Geometry check sheet. Reference: the model listing, model coordinates, mm. A direction names the side the tool comes from. Coordinates: 2 decimals unless noted, no trailing zeros. Order: outer loops, then holes, each group sorted by start corner. A loop starts at its lowest first (then second) coordinate and runs counter-clockwise, first axis right, second up. Notation, with made-up numbers: (59.25, 45.25) - (103.25, 45.25) arc R25 cw to (103.25, 78.25) - close; hole circle Ø2 at (-34.75, -15.75). An arc over 180 degrees is marked (long way). One line per item, written item: value. Start each with the question number.
Autodesk Inventor part; units mm, degrees
ref_plane "YZ Plane" through (0, 0, 0) normal (1, 0, 0) x (0, 1, 0)
ref_plane "XZ Plane" through (0, 0, 0) normal (0, 1, 0) x (-1, 0, 0)
ref_plane "XY Plane" through (0, 0, 0) normal (0, 0, 1) x (1, 0, 0)
sketch "スケッチ1" plane through (0, 0, 0) normal (0, 0, 1) x (1, 0, 0)
  line L0 (-59.5, -21.75) -> (59.5, -21.75) construction
  line L1 (59.5, -21.75) -> (59.5, 21.75) construction
  line L2 (59.5, 21.75) -> (-59.5, 21.75) construction
  line L3 (-59.5, 21.75) -> (-59.5, -21.75) construction
  line L4 (-59.5, -21.75) -> (59.5, 21.75) construction
  line L5 (59.5, -21.75) -> (-59.5, 21.75) construction
  line L6 (-54.5, -16.75) -> (54.5, -16.75) construction
  line L7 (54.5, -16.75) -> (54.5, 16.75) construction
  line L8 (54.5, 16.75) -> (-54.5, 16.75) construction
  line L9 (-54.5, 16.75) -> (-54.5, -16.75) construction
  line L10 (-54.5, -16.75) -> (54.5, 16.75) construction
  line L11 (54.5, -16.75) -> (-54.5, 16.75) construction
  line L12 (-33.05, 11.05) -> (-27.95, 11.05)
  line L13 (-27.95, 11.05) -> (-27.95, -4.05)
  line L14 (-27.95, -4.05) -> (-33.05, -4.05)
  line L15 (-33.05, -4.05) -> (-33.05, 11.05)
  line L16 (-28, 11) -> (-33, 11) construction
  line L17 (-33, 11) -> (-33, -4) construction
  line L18 (-33, -4) -> (-28, -4) construction
  line L19 (-28, -4) -> (-28, 11) construction
  line L20 (-30.5, 11) -> (-30.5, -4) construction
  line L21 (-33, 21) -> (-28, 21) construction
  line L22 (-28, 21) -> (-28, -14) construction
  line L23 (-28, -14) -> (-33, -14) construction
  line L24 (-33, -14) -> (-33, 21) construction
  circle A0 centre (-30.5, 17) radius 1.55
  circle A1 centre (-30.5, -10) radius 1.55
  circle A2 centre (-33.05, 10) radius 1.05
  circle A3 centre (-27.95, 10) radius 1.05
  circle A4 centre (-33.05, -3) radius 1.05
  circle A5 centre (-27.95, -3) radius 1.05
  line L25 (0, 0) -> (0, 16.75) construction
  line L26 (0, 0) -> (54.5, 0) construction
  circle A6 centre (30.5, 17) radius 1.55
  circle A7 centre (30.5, -10) radius 1.55
  circle A8 centre (27.95, 10) radius 1.05
  circle A9 centre (33.05, 10) radius 1.05
  circle A10 centre (27.95, -3) radius 1.05
  circle A11 centre (33.05, -3) radius 1.05
  line L27 (33.05, 11.05) -> (27.95, 11.05)
  line L28 (27.95, 11.05) -> (27.95, -4.05)
  line L29 (27.95, -4.05) -> (33.05, -4.05)
  line L30 (33.05, -4.05) -> (33.05, 11.05)
  line L31 (-59.5, 11.75) -> (-64.5, 11.75)
  line L32 (-64.5, 11.75) -> (-64.5, -11.75)
  line L33 (-64.5, -11.75) -> (-59.5, -11.75)
  line L34 (-59.5, 13.85) -> (-59.5, 21.75)
  line L35 (-59.5, 21.75) -> (-21.6, 21.75)
  line L36 (-19.5, 21.75) -> (-19.5, 26.75)
  line L37 (-19.5, 26.75) -> (19.5, 26.75)
  line L38 (19.5, 26.75) -> (19.5, 21.75)
  line L39 (21.6, 21.75) -> (59.5, 21.75)
  line L40 (59.5, 21.75) -> (59.5, 13.85)
  line L41 (59.5, 11.75) -> (64.5, 11.75)
  line L42 (64.5, 11.75) -> (64.5, -11.75)
  line L43 (64.5, -11.75) -> (59.5, -11.75)
  line L44 (-59.5, -13.85) -> (-59.5, -21.75)
  line L45 (-59.5, -21.75) -> (59.5, -21.75)
  line L46 (59.5, -21.75) -> (59.5, -13.85)
  arc A12 (-59.5, 11.75) -> (-59.5, 13.85) centre (-59.5, 12.8) ccw
  arc A13 (-59.5, -13.85) -> (-59.5, -11.75) centre (-59.5, -12.8) ccw
  line L47 (0, 0) -> (-54.5, 0) construction
  arc A14 (59.5, -11.75) -> (59.5, -13.85) centre (59.5, -12.8) ccw
  arc A15 (59.5, 13.85) -> (59.5, 11.75) centre (59.5, 12.8) ccw
  arc A16 (-21.6, 21.75) -> (-19.5, 21.75) centre (-20.55, 21.75) ccw
  arc A17 (19.5, 21.75) -> (21.6, 21.75) centre (20.55, 21.75) ccw
  line L48 (-56.8855, 19.3) -> (-54.5, 19.3) construction
  line L49 (-54.5, 19.3) -> (-54.5, 16.2) construction
  line L50 (-54.5, 16.2) -> (-56.8855, 16.2) construction
  line L51 (-56.8855, 16.2) -> (-56.8855, 19.3) construction
  line L52 (-54.5, 17.75) -> (-56.8855, 17.75) construction
  line L53 (-53.05, 22.7202) -> (-49.95, 22.7202) construction
  line L54 (-49.95, 22.7202) -> (-49.95, 16.75) construction
  line L55 (-49.95, 16.75) -> (-53.05, 16.75) construction
  line L56 (-53.05, 16.75) -> (-53.05, 22.7202) construction
  line L57 (-51.5, 22.7202) -> (-51.5, 16.75) construction
  point P0 (-30.5, -14)
  dimension "d10" = 2.1
  dimension "d0" = 33.5
  dimension "d1" = 5
  dimension "d2" = 109
  dimension "d3" = 5
  dimension "d4" = 0.05
  dimension "d5" = 35
  dimension "d6" = 27
  dimension "d7" = 5
  dimension "d11" = 33
  dimension "d12" = 3.1
  dimension "d13" = 1.05
  dimension "d14" = 5
  dimension "d15" = 4
  dimension "d16" = 3.1
  dimension "d17" = 10
  dimension "d18" = 5
  dimension "d19" = 8
  dimension "d20" = 5
  dimension "d21" = 40
  dimension "d22" = 5
  dimension "d50" = 4
  dimension "d51" = 10
  dimension "d52" = 17
  dimension "d53" = 10
extrude "押し出し1" add sketch "スケッチ1" along normal blind 5
sketch "スケッチ2" plane through (0, 0, 5) normal (0, 0, 1) x (1, 0, 0)
  circle A0 centre (30.5, -10) radius 1.55
  circle A1 centre (30.5, 17) radius 1.55
  circle A2 centre (-30.5, -10) radius 1.55
  circle A3 centre (-30.5, 17) radius 1.55
  point P0 (0, 0)
hole "穴1" at (-30.5, 17, 5) at (-30.5, -10, 5) at (30.5, 17, 5) at (30.5, -10, 5) direction (0, 0, -1) diameter 6 depth 3
sketch "スケッチ3" plane through (59.5, -21.75, 0) normal (1, 0, 0) x (0, 0, -1)
  line L0 (0, 0) -> (-5, 0)
  line L1 (0, 43.5) -> (-5, 43.5)
  point P0 (0, 21.75)
  point P1 (-2.5, 4)
  point P2 (-2.5, 39.5)
  point P3 (-2.5, 0)
  dimension "d32" = 4
  dimension "d33" = 4
hole "穴2" at (59.5, -17.75, 2.5) at (59.5, 17.75, 2.5) direction (-1, 0, 0) diameter 2.459 depth 2.5
mirror "ミラー1" about plane through (0, 0, 0) normal (1, 0, 0) of "穴2"
sketch "スケッチ5" plane through (0, 0, 5) normal (0, 0, 1) x (1, 0, 0)
  line L0 (27.95, -1.95) -> (27.95, 8.95)
  line L1 (-33.05, -1.95) -> (-33.05, 8.95)
  line L2 (-27.95, 8.95) -> (-27.95, -1.95)
  line L3 (-59.5, -21.75) -> (59.5, -21.75)
  line L4 (19.5, 26.75) -> (-19.5, 26.75)
  line L5 (-21.6, 21.75) -> (-59.5, 21.75)
  line L6 (-59.5, 21.75) -> (-59.5, 13.85)
  line L7 (-52.5, 14.75) -> (-38, 14.75)
  line L8 (-38, 14.75) -> (-38, -14.75)
  line L9 (-38, -14.75) -> (-52.5, -14.75)
  line L10 (-52.5, -14.75) -> (-52.5, 14.75)
  line L11 (38, 14.75) -> (52.5, 14.75)
  line L12 (52.5, 14.75) -> (52.5, -14.75)
  line L13 (52.5, -14.75) -> (38, -14.75)
  line L14 (38, -14.75) -> (38, 14.75)
  line L15 (-23, 16.75) -> (-23, -9.0978)
  line L16 (-23, -9.0978) -> (20.2083, 16.75)
  line L17 (20.2083, 16.75) -> (-23, 16.75)
  line L18 (23, 9.0978) -> (23, -16.75)
  line L19 (23, -16.75) -> (-20.2083, -16.75)
  line L20 (-20.2083, -16.75) -> (23, 9.0978)
  line L21 (-33, 9.2736) -> (-28, 9.2736) construction
  line L22 (-28, 9.2736) -> (-28, -5.1442) construction
  line L23 (-28, -5.1442) -> (-33, -5.1442) construction
  line L24 (-33, -5.1442) -> (-33, 9.2736) construction
  line L25 (0, 0) -> (0, 26.75) construction
  line L26 (28, 10.3975) -> (29.3974, 10.3975) construction
  line L27 (29.3974, 10.3975) -> (29.3974, -4.5864) construction
  line L28 (29.3974, -4.5864) -> (28, -4.5864) construction
  line L29 (28, -4.5864) -> (28, 10.3975) construction
  line L30 (28, 16.75) -> (-28, -16.75) construction
  line L31 (-28, 16.75) -> (28, 16.75) construction
  line L32 (28, 16.75) -> (28, -16.75) construction
  line L33 (28, -16.75) -> (-28, -16.75) construction
  line L34 (-28, -16.75) -> (-28, 16.75) construction
  line L35 (59.5, 21.75) -> (21.6, 21.75)
  dimension "d54" = 7
  dimension "d55" = 7
  dimension "d56" = 7
  dimension "d57" = 0.05
  dimension "d58" = 5
  dimension "d59" = 0.05
  dimension "d60" = 5
  dimension "d62" = 5
  dimension "d63" = 0.05
  dimension "d64" = 8
  dimension "d68" = 5
extrude "押し出し2" cut sketch "スケッチ5" against normal blind 10
fillet "フィレット1" radius 3 14 edges at (-38, 14.75, 2.5) (-52.5, 14.75, 2.5) (-52.5, -14.75, 2.5) (-38, -14.75, 2.5) (-23, -9.0978, 2.5) (-23, 16.75, 2.5) (20.2083, 16.75, 2.5) (23, 9.0978, 2.5) (-20.2083, -16.75, 2.5) (23, -16.75, 2.5) (38, -14.75, 2.5) (52.5, -14.75, 2.5) (52.5, 14.75, 2.5) (38, 14.75, 2.5)
equation "\"d20\" = d18"
equation "\"d53\" = d51"
equation "\"d56\" = d55"
equation "\"d59\" = d57"
equation "\"d60\" = d58"
properties part number "コックピット_サブフレーム_1_3" material "アセタール樹脂、黒"
Q1. Set-up check for faces 1 (the cylindrical face through (-21.44, -6.44, 2.46)), 2 (the cylindrical face through (58.23, 16.53, 2.66)), 3 (the cylindrical face through (31.65, -12.77, 3.48)): record each of +Z, -Z, +X, -X, +Y, -Y from which the full face is reachable in a straight line by a thin tool's end or side.
Q2. Cross-section at A-A, the plane x = -46.5. Enter the section's corners in (y, z), and give its area (3 significant figures).
Q3. Release check for a two-part mould opening along Z. For faces 4 (the flat face through (-23, 5, 3)), 5 (the flat face through (-29, -11, 2)), 6 (the cylindrical face through (-58.23, -16.53, 2.66)), 7 (the flat face through (57, 18, 3)) record: released by +Z, released by -Z, zero draft, split by the parting line, or undercut.
Q4. Gauge pin test, flat ends, axial feed: P1, Ø2.5, axis at x = 46.5, z = 1.5, coming from the +Y side; P2, Ø1.2, axis at y = 17.5, z = 2.5, coming from the -X side; P3, Ø3, axis at x = 30.5, y = 16.5, coming from the +Z side. Record the tip position at first contact, or that the pin passes through.
Q5. Material ranges on probe 1 along Y at (x, z) = (58.3, 2.5); probe 2 along Y at (x, z) = (-30.5, 0.8); probe 3 along Y at (x, z) = (-30.5, 3.05), recorded low to high.
Q6. Cross-section at B-B, the plane y = -10. Count the separate pieces of the cut face and the enclosed holes in it, and give its area (3 significant figures).
Q7. Cross-section at C-C, the plane x = -30.5. Enter the section's corners in (y, z), and give its area (3 significant figures).
Check result:
1. face 1: +Z, -Z
1. face 2: +X
1. face 3: +Z
2. outline: (-21.75, 0) - (-14.75, 0) - (-14.75, 5) - (-21.75, 5) - close; (14.75, 0) - (21.75, 0) - (21.75, 5) - (14.75, 5) - close
2. area: 70.0 mm2
3. face 4: zero draft
3. face 5: released by +Z
3. face 6: undercut
3. face 7: undercut
4. P1: stops at y = 21.75
4. P2: stops at x = -57
4. P3: stops at z = 2
5. probe 1: y = -21.75 to -18.98, -16.52 to 16.52, 18.98 to 21.75
5. probe 2: y = -21.75 to -11.55, -8.45 to -4.05, 11.05 to 15.45, 18.55 to 21.75
5. probe 3: y = -21.75 to -13, -7 to -4.05, 11.05 to 14, 20 to 21.75
6. separate pieces: 6
6. enclosed holes: 0
6. area: 292 mm2
7. outline: (-21.75, 0) - (-11.55, 0) - (-11.55, 2) - (-13, 2) - (-13, 5) - (-21.75, 5) - close; (-8.45, 0) - (-4.05, 0) - (-4.05, 5) - (-7, 5) - (-7, 2) - (-8.45, 2) - close; (11.05, 0) - (15.45, 0) - (15.45, 2) - (14, 2) - (14, 5) - (11.05, 5) - close; (18.55, 0) - (21.75, 0) - (21.75, 5) - (20, 5) - (20, 2) - (18.55, 2) - close
7. area: 93.6 mm2
